from build123d import *

# Parameters (mm, degrees)
SKETCH1_W           = 20
SKETCH1_H           = 20
BOSS_EXTRUDE1_DEPTH = 0.4
SKETCH2_R           = 1.6
CUT_EXTRUDE1_DEPTH  = 0.4


with BuildPart() as part:
    # Sketch1 → Boss-Extrude1 (new body)
    with BuildSketch(Plane(origin=(0, 0, 0), x_dir=(0, 0, -1), z_dir=(1, 0, 0))):
        with Locations((-132.306860457, -13.392602836)):
            Rectangle(SKETCH1_W, SKETCH1_H)
    extrude(amount=BOSS_EXTRUDE1_DEPTH)

    # Sketch2 → Cut-Extrude1 (cut)
    with BuildSketch(Plane.ZY):
        with Locations((126.306860457, -8.392602836)):
            Circle(SKETCH2_R)
        with Locations((126.306860457, -16.392602836)):
            Circle(SKETCH2_R)
        with Locations((135.306860457, -8.392602836)):
            Circle(SKETCH2_R)
        with Locations((135.306860457, -16.392602836)):
            Circle(SKETCH2_R)
    extrude(amount=-CUT_EXTRUDE1_DEPTH, mode=Mode.SUBTRACT)


solid = part.part
For this review, take the finished solid that the model builds, in its own axes (mm). Round coordinates to 2 decimals unless told otherwise and drop trailing zeros. Write each loop counter-clockwise with the first axis right and the second up, starting at its lowest first coordinate (ties: lowest second). Pieces come first, ordered by that corner, then holes. Notation, with made-up numbers: (71, -4) -> (85, -4) arc R24 ccw to (85, 13) -> close; hole circle Ø4 at (-16, 14.5). An arc over 180 degrees is marked (long way). Put each result on its own line as item: value.
Q1. Clearance check with a flat-ended pin moving along its axis: pin 1 Ø10 at (y, z) = (-12, 128) entering from -X. State where the tip first meets the part, or that it passes through.
Determined:
pin 1: stops at x = 0
Q2. Consider section B-B on x = 0.3. State the section outline as (y, z) points.
Determined:
outline: (-23.39, 122.31) -> (-3.39, 122.31) -> (-3.39, 142.31) -> (-23.39, 142.31) -> close; hole circle Ø3.2 at (-16.39, 126.31); hole circle Ø3.2 at (-16.39, 135.31); hole circle Ø3.2 at (-8.39, 126.31); hole circle Ø3.2 at (-8.39, 135.31)
Q3. Consider section A-A on z = 135.25. State the section outline as (x, y) points.
Determined:
outline: (0, -23.39) -> (0.4, -23.39) -> (0.4, -17.99) -> (0, -17.99) -> close; (0, -14.79) -> (0.4, -14.79) -> (0.4, -9.99) -> (0, -9.99) -> close; (0, -6.79) -> (0.4, -6.79) -> (0.4, -3.39) -> (0, -3.39) -> close
Q4. The part is to be moulded in two halves that separate along Z. For faces 1 (the cylindrical face through (0.197, -15.912, 136.833)), 2 (the flat face through (0.4, -13, 132)), 3 (the cylindrical face through (0.197, -7.912, 136.833)), say which applies: released by +Z, released by -Z, zero draft, split by the parting line, or undercut.
Determined:
face 1: undercut
face 2: zero draft
face 3: undercut
Q5. To check wall thickness, follow L1, parallel to Y at x = 0.1, z = 126; L2, parallel to Y at x = 0.15, z = 125; L3, parallel to Z at x = 0.2, y = -17.5. State the ranges of each line that lie inside material, in increasing order. Write a range as [from, to].
Determined:
L1: y = [-23.39, -17.96], [-14.82, -9.96], [-6.82, -3.39]
L2: y = [-23.39, -17.32], [-15.47, -9.32], [-7.47, -3.39]
L3: z = [122.31, 125.15], [127.46, 134.15], [136.46, 142.31]
Q6. Consider section C-C on y = -17.75. State the section outline as (x, z) points, and give its area (3 significant figures).
Determined:
outline: (0, 122.31) -> (0.4, 122.31) -> (0.4, 125.46) -> (0, 125.46) -> close; (0, 127.15) -> (0.4, 127.15) -> (0.4, 134.46) -> (0, 134.46) -> close; (0, 136.15) -> (0.4, 136.15) -> (0.4, 142.31) -> (0, 142.31) -> close
area: 6.64 mm^2
